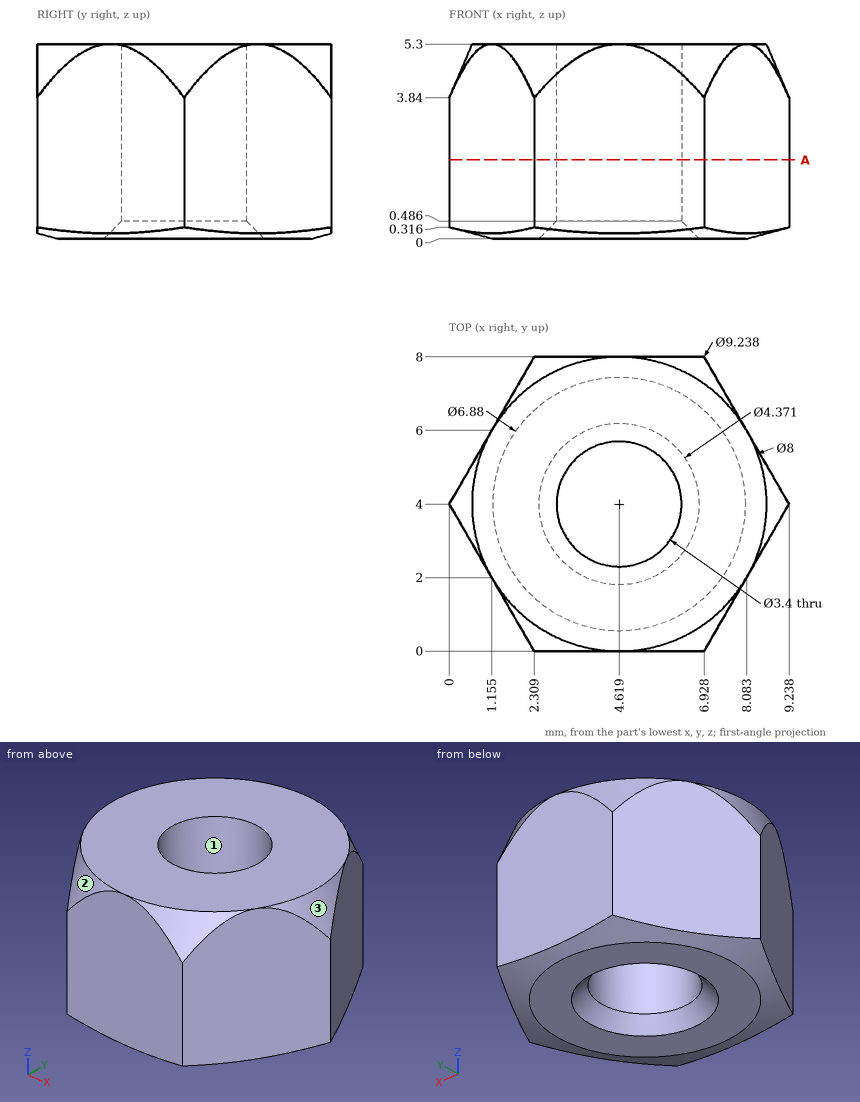
Study the drawing (mm; zero at the part's minimum x, y, z) and answer. Coordinates: 2 decimals unless noted, no trailing zeros. Loops run counter-clockwise (first coordinate to the right, second up) from the corner with the lowest first, then second, coordinate; pieces in that order, holes last. Notation, with made-up numbers: M 69,11.5 L 92,11.5 A27 cw 92,40.5 Z; hole C 50.25,63.5 d4. An arc over 180 degrees is marked long. Answer in a Markdown table with one row per item.
1) Determine the mould class of the marked faces 1, 2 and 3 for opening direction X: released by +X, released by -X, zero draft, split by the parting line, or undercut.
Answers below:
| item | result |
|---|---|
| face 1 | undercut |
| face 2 | released by -X |
| face 3 | released by +X |
2) Given pin 1 (2 mm diameter, centred on y = 6.5, z = 2, fed in from -X) (1 decimal), flat-ended and moving along its own axis, determine where the tip first touches the part or whether it passes through.
Answers below:
| item | result |
|---|---|
| pin 1 | x = 0.9 |
3) Find the intervals of material crossed by probe 1 along X at (y, z) = (2, 3.4) (1 decimal); probe 2 along Y at (x, z) = (3.25, 1.3) (1 decimal); probe 3 along X at (y, z) = (2.75, 2.2) (1 decimal), in increasing order.
Answers below:
| item | result |
|---|---|
| probe 1 | 1.2 to 8.1 |
| probe 2 | 0 to 3, 5 to 8 |
| probe 3 | 0.7 to 3.5, 5.8 to 8.5 |
4) Find section A-A (z = 2.15). Determine the outline of the cut face in (x, y).
Answers below:
| item | result |
|---|---|
| outline | M 0,4 L 2.31,0 L 6.93,0 L 9.24,4 L 6.93,8 L 2.31,8 Z; hole C 4.62,4 d3.4 |
